```python
from build123d import *

# Parameters (mm, degrees)
SKETCH3_R               = 29.21
SKETCH3_R_2             = 6.35
BOSS_EXTRUDE1_DEPTH     = 76.2
CUT_EXTRUDE1_DEPTH      = 87.676918496
CUT_EXTRUDE1_DEPTH_BACK = 87.676918496
SKETCH4_W               = 68.58
SKETCH4_H               = 78.74
SHELL4_START            = 3.81
SHELL4_DEPTH            = 68.58
CUT_EXTRUDE2_DEPTH      = 3.81


# Read off the part's stored shape, not the designer's step: Shell4
with BuildPart() as part:
    # Sketch3 → Boss-Extrude1 (new body)
    with BuildSketch(Plane(origin=(0, 0, 0), x_dir=(0, 0, -1), z_dir=(1, 0, 0))):
        with Locations(Location((0, 0, 0), (0, 0, 180))):
            Circle(SKETCH3_R)
        with Locations(Location((0, 0, 0), (0, 0, 180))):
            Circle(SKETCH3_R_2, mode=Mode.SUBTRACT)
    extrude(amount=BOSS_EXTRUDE1_DEPTH)

    # Sketch4 → Cut-Extrude1 (cut, two sides: drawn at the far end of the back side and taken through both)
    with BuildSketch(Plane.XY.offset(-CUT_EXTRUDE1_DEPTH_BACK)):
        with Locations((38.1, 29.21)):
            Rectangle(SKETCH4_W, SKETCH4_H)
    extrude(amount=CUT_EXTRUDE1_DEPTH + CUT_EXTRUDE1_DEPTH_BACK, mode=Mode.SUBTRACT)

    # Shell4 outline → Shell4 (cut)
    with BuildSketch(Plane.YZ.offset(SHELL4_START)):
        with BuildLine():
            ThreePointArc((-10.16, 23.27948453), (-25.4, 0), (-10.16, -23.27948453))
            Line((-10.16, -23.27948453), (-10.16, 23.27948453))
        make_face()
    extrude(amount=SHELL4_DEPTH, mode=Mode.SUBTRACT)

    # Sketch5 → Cut-Extrude2 (cut)
    with BuildSketch(Plane.ZY):
        Polygon((24.13, 10.16), (19.730590949, 7.62), (24.13, 5.08), (19.730590949, 2.54), (24.13, 0), (19.730590949, -2.54), (24.13, -5.08), (19.730590949, -7.62), (24.13, -10.16), (29.21, -10.16), (29.21, 10.16), align=None)
        Polygon((-29.21, 10.16), (-24.13, 10.16), (-19.730590949, 7.62), (-24.13, 5.08), (-19.730590949, 2.54), (-24.13, 0), (-19.730590949, -2.54), (-24.13, -5.08), (-19.730590949, -7.62), (-24.13, -10.16), (-29.21, -10.16), align=None)
    extrude(amount=-CUT_EXTRUDE2_DEPTH, mode=Mode.SUBTRACT)


solid = part.part
```
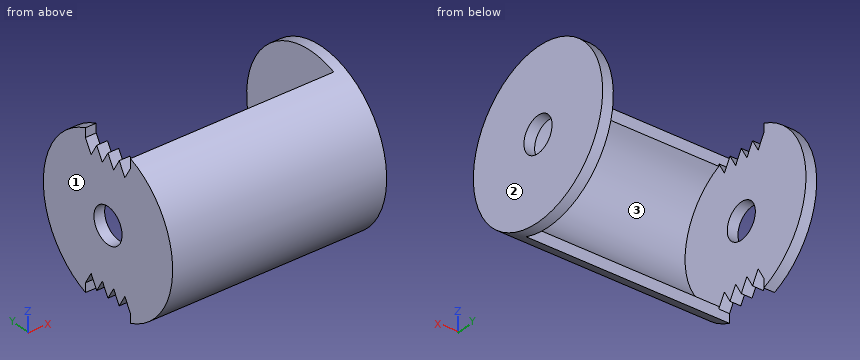
The listing builds one solid part. Answer for the finished solid, in the listing's coordinates (mm). Face numbers are marked on the shaded views. Coordinates: 2 decimals unless noted, no trailing zeros. Write each loop counter-clockwise with the first axis right and the second up, starting at its lowest first coordinate (ties: lowest second). Pieces come first, ordered by that corner, then holes. Notation, with made-up numbers: M 56,-25.75 L 100,-25.75 A15 ccw 100,3.25 Z; hole C 66.5,12.5 d5. An arc over 180 degrees is marked long. Use a Markdown table: item, result. Add a question column.
1. Given P1, Ø10, axis at x = 36.5, y = -15, coming from the +Z side; P2, Ø2.5, axis at x = 2, z = -26, coming from the -Y side; P3, Ø10, axis at x = 9.5, z = 7, coming from the -Y side; P4, Ø10, axis at y = 0, z = 0, coming from the -X side, each flat-ended and moving along its own axis, determine where each tip first touches the part or whether it passes through.
2. For a pull along X with two mould halves and no side action, classify the marked faces 1, 2 and 3 as +X half, -X half, draft (parallel to the pull), parting line (faces both ways), or undercut.
3. Straight lines are drawn through the part: line 1 along Y through (x, z) = (75.2, 0); line 2 along X through (y, z) = (11, -9.5); line 3 along Z through (x, y) = (25, -12). For each, find the intervals that lie inside material, in ascending order. Write a range as [from, to].
4. Section D-D (z = 25.5) is taken. Give the vertices of the cut face in (x, y), plus the area to 3 significant figures.
5. Section C-C (z = -21) is taken. Give the vertices of the cut face in (x, y).
6. Section A-A (z = 0) is taken. Give the vertices of the cut face in (x, y).
7. Section B-B (y = 18) is taken. Give the vertices of the cut face in (x, z), plus the area to 3 significant figures.
Data:
| question | item | result |
|---|---|---|
| 1 | P1 | stops at z = 27.39 |
| 1 | P2 | stops at y = -15.51 |
| 1 | P3 | stops at y = -29.14 |
| 1 | P4 | passes through |
| 2 | face 1 | -X half |
| 2 | face 2 | +X half |
| 2 | face 3 | undercut |
| 3 | line 1 | y = [-29.21, -6.35], [6.35, 29.21] |
| 3 | line 2 | x = [0, 3.81], [72.39, 76.2] |
| 3 | line 3 | z = [-26.63, -22.39], [22.39, 26.63] |
| 4 | outline | M 0,-14.25 L 76.2,-14.25 L 76.2,14.25 L 72.39,14.25 L 72.39,-10.16 L 0,-10.16 Z; M 0,10.16 L 3.81,10.16 L 3.81,14.25 L 0,14.25 Z |
| 4 | area | 420 mm2 |
| 5 | outline | M 0,-20.3 L 76.2,-20.3 L 76.2,20.3 L 72.39,20.3 L 72.39,-14.29 L 3.81,-14.29 L 3.81,-8.35 L 0,-8.35 Z; M 0,-6.89 L 3.81,-6.89 L 3.81,-3.27 L 0,-3.27 Z; M 0,-1.81 L 3.81,-1.81 L 3.81,1.81 L 0,1.81 Z; M 0,3.27 L 3.81,3.27 L 3.81,6.89 L 0,6.89 Z; M 0,8.35 L 3.81,8.35 L 3.81,20.3 L 0,20.3 Z |
| 6 | outline | M 0,-29.21 L 76.2,-29.21 L 76.2,-6.35 L 72.39,-6.35 L 72.39,-25.4 L 3.81,-25.4 L 3.81,-6.35 L 0,-6.35 Z; M 0,6.35 L 3.81,6.35 L 3.81,29.21 L 0,29.21 Z; M 72.39,6.35 L 76.2,6.35 L 76.2,29.21 L 72.39,29.21 Z |
| 7 | outline | M 0,-23 L 3.81,-23 L 3.81,23 L 0,23 Z; M 72.39,-23 L 76.2,-23 L 76.2,23 L 72.39,23 Z |
| 7 | area | 351 mm2 |
